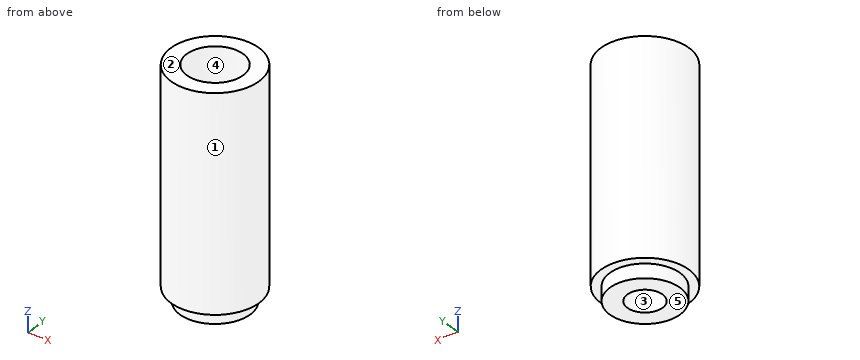
```python
from build123d import *

# Parameters (mm, degrees)
SKETCH_1_R            = 12.5
EXTRUDE_1_DEPTH       = 60
SKETCH_2_R            = 10
EXTRUDE_2_DEPTH       = 4
OTHER_START           = 45
OTHER_1_OUTLINE_R     = 8
OTHER_1_DEPTH         = 15
M10X1_251_D           = 8.8
M10X1_251_DEPTH       = 40
M10X1_251_CBORE_D     = 10
M10X1_251_CBORE_DEPTH = 20
M10X1_251_TIP         = 2.643786724


# Read off the part's stored shape, not the designer's step: Полость1
with BuildPart() as part:
    # Эскиз1 → Бобышка-Вытянуть1 (new body)
    with BuildSketch(Plane.XY):
        with Locations((51.75, 69.5)):
            Circle(SKETCH_1_R)
    extrude(amount=EXTRUDE_1_DEPTH)

    # Эскиз2 → Бобышка-Вытянуть2 (add)
    with BuildSketch(Plane(origin=(0, 0, 0), x_dir=(-1, 0, 0), z_dir=(0, 0, -1))):
        with Locations((-51.75, 69.5)):
            Circle(SKETCH_2_R)
    extrude(amount=EXTRUDE_2_DEPTH)

    # Полость1 outline → Полость1 (cut)
    with BuildSketch(Plane.XY.offset(OTHER_START)):
        with Locations((51.75, 69.5)):
            Circle(OTHER_1_OUTLINE_R)
    extrude(amount=OTHER_1_DEPTH, mode=Mode.SUBTRACT)

    # Отверстие обработанное метчиком M10x1.251
    with Locations(Plane(origin=(0, 0, -4), x_dir=(-1, 0, 0), z_dir=(0, 0, -1))):
        with Locations((-51.75, 69.5)):
            CounterBoreHole(M10X1_251_D / 2, M10X1_251_CBORE_D / 2, M10X1_251_CBORE_DEPTH, depth=M10X1_251_DEPTH)
            with Locations((0, 0, -(M10X1_251_DEPTH + M10X1_251_TIP / 2))):  # 118° drill point
                Cone(0, M10X1_251_D / 2, M10X1_251_TIP, mode=Mode.SUBTRACT)


solid = part.part
```
Verification items for the finished model (mm, model axes). Face numbers are marked on the shaded views. A direction names the side the tool comes from. Round coordinates to 2 decimals unless told otherwise and drop trailing zeros. Order: outer loops, then holes, each group sorted by start corner. A loop starts at its lowest first (then second) coordinate and runs counter-clockwise, first axis right, second up. Notation, with made-up numbers: (66, 47.5) -> (93, 47.5) arc R31 ccw to (93, 75.5) -> close; hole circle Ø11 at (45.5, 44.25). An arc over 180 degrees is marked (long way). Put each result on its own line as item: value. Start each with the question number.
(1) Section check C-C (y = 78.5). Enter the section's corners in (x, z).
(2) Depth check by flat-ended pin: pin 1 Ø3 at (x, z) = (54.5, 19.5) entering from -Y; pin 2 Ø1 at (y, z) = (63, 34) entering from -X; pin 3 Ø7.5 at (x, y) = (50.5, 68) entering from -Z; pin 4 Ø8 at (y, z) = (76.5, 35.5) entering from +X. Enter the tip coordinate at first touch or a pass-through.
(3) Draft check along X on the marked faces 1, 2 and 3. Enter one of: +X half, -X half, draft (parallel to the pull), parting line (faces both ways), or undercut.
(4) Section check A-A (z = 46.5). Enter the section's corners in (x, y).
(5) Section check B-B (x = 60.5). Enter the section's corners in (y, z), then the cut area to 3 significant figures.
(6) Tool access check on the marked faces 4 and 5. Record the directions out of +Z, -Z, +X, -X, +Y, -Y that give a thin tool (end or side, any length) a straight path to the whole face; none if there is none.
(7) Material ranges on line 1 along Y through (x, z) = (51.75, 31.25); line 2 along Y through (x, z) = (51.75, 10.5); line 3 along Z through (x, y) = (54.5, 79.5), recorded low to high.
(8) Section check D-D (y = 63.5). Enter the section's corners in (x, z).
Completed:
1. outline: (43.08, 0) -> (47.39, 0) -> (47.39, -4) -> (56.11, -4) -> (56.11, 0) -> (60.42, 0) -> (60.42, 60) -> (43.08, 60) -> close
2. pin 1: stops at y = 57.06
2. pin 2: stops at x = 40.78
2. pin 3: stops at z = -4
2. pin 4: stops at x = 63.88
3. face 1: parting line
3. face 2: draft
3. face 3: undercut
4. outline: circle Ø25 at (51.75, 69.5); hole circle Ø16 at (51.75, 69.5)
5. outline: (60.57, 0) -> (64.66, 0) -> (64.66, -4) -> (74.34, -4) -> (74.34, 0) -> (78.43, 0) -> (78.43, 60) -> (60.57, 60) -> close
5. area: 1,110 mm2
6. face 4: +Z
6. face 5: -Z, +X, -X, +Y, -Y
7. line 1: y = 57 to 65.1, 73.9 to 82
7. line 2: y = 57 to 64.5, 74.5 to 82
7. line 3: z = 0 to 60
8. outline: (40.78, 0) -> (43.75, 0) -> (43.75, -4) -> (59.75, -4) -> (59.75, 0) -> (62.72, 0) -> (62.72, 60) -> (57.04, 60) -> (57.04, 45) -> (46.46, 45) -> (46.46, 60) -> (40.78, 60) -> close
